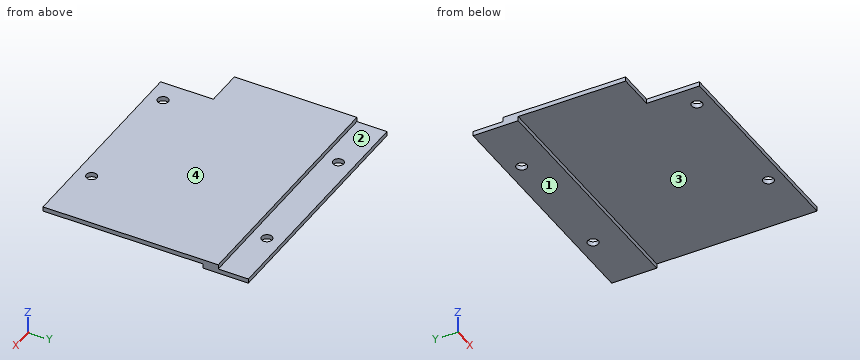
Solid Edge part; units mm, degrees
sketch "Sketch1" plane through (0, 0, 0) normal (0, 0, 1) x (1, 0, 0)
  line L0 (-82.5, -68.15) -> (82.5, -68.15)
  line L1 (82.5, -68.15) -> (82.5, 68.15)
  line L2 (82.5, 68.15) -> (-82.5, 68.15)
  line L3 (-82.5, 68.15) -> (-82.5, -68.15)
  dimension "D1" = 82.5
  dimension "D2" = 82.5
extrude "Extrusionsausprägung_1" add sketch "Sketch1" along normal blind 3
sketch "Sketch2" plane through (0, 0, 3) normal (0, 0, 1) x (1, 0, 0)
  circle A0 centre (-42.5, 58.15) radius 3.5
  circle A1 centre (42.5, 58.15) radius 3.5
  circle A2 centre (42.5, -58.15) radius 3.5
  circle A3 centre (-42.5, -58.15) radius 3.5
  dimension "D1" = 42.5
extrude "Extrusionsausschnitt_1" cut sketch "Sketch2" against normal blind 245.2559
sketch "Sketch3" plane through (0, 0, 3) normal (0, 0, 1) x (1, 0, 0)
  line L0 (-82.5, -68.15) -> (-57.5, -68.15)
  line L1 (-57.5, -68.15) -> (-57.5, -33.15)
  line L2 (-57.5, -33.15) -> (-82.5, -33.15)
  line L3 (-82.5, -33.15) -> (-82.5, -68.15)
  dimension "D1" = 57.5
  dimension "D2" = 57.5
extrude "Cutout1" cut sketch "Sketch3" against normal through all
sketch "Sketch4" plane through (0, 0, 0) normal (0, 0, -1) x (-1, 0, 0)
  line L0 (-82.5, 68.15) -> (82.5, 68.15)
  line L1 (82.5, 68.15) -> (82.5, 38.15)
  line L2 (82.5, 38.15) -> (-82.5, 38.15)
  line L3 (-82.5, 38.15) -> (-82.5, 68.15)
  dimension "D1" = 82.5
  dimension "D2" = 82.5
extrude "Extrusionsausprägung_2" add sketch "Sketch4" along normal blind 3
sketch "Sketch5" plane through (0, 0, 3) normal (0, 0, 1) x (1, 0, 0)
  circle A0 centre (-42.5, 58.15) radius 3.5
  circle A1 centre (42.5, 58.15) radius 3.5
extrude "Cutout2" cut sketch "Sketch5" against normal through all
sketch "Sketch6" plane through (-82.5, 17.5, 0) normal (-1, 0, 0) x (0, 1, 0)
  line L0 (50.65, 0) -> (30.65, 0)
  line L1 (30.65, 0) -> (30.65, -3)
  line L2 (30.65, -3) -> (50.65, -3)
  line L3 (50.65, -3) -> (50.65, 0)
  dimension "D1" = 30.65
  dimension "D2" = 50.65
extrude "Cutout3" cut sketch "Sketch6" against normal through all
properties material "Nylon, allgemein"
Work out the finished part from the listing and answer in its coordinate system (mm). Face numbers are marked on the shaded views. A direction names the side the tool comes from. Round coordinates to 2 decimals unless told otherwise and drop trailing zeros. Loops run counter-clockwise (first coordinate to the right, second up) from the corner with the lowest first, then second, coordinate; pieces in that order, holes last. Notation, with made-up numbers: (12, 24.25) -> (59, 24.25) arc R18 cw to (59, 49.25) -> close; hole circle Ø7 at (61, -33.5). An arc over 180 degrees is marked (long way). Use one line per item in the form item = value.
(1) For a pull along Z with two mould halves and no side action, classify the marked faces 3 and 4 as released by +Z, released by -Z, zero draft, split by the parting line, or undercut.
Answer list:
face_3 = released by -Z
face_4 = released by +Z
(2) Find section A-A on y = -58.15. Give the vertices of the cut face in (x, z).
Answer list:
outline = (-57.5, 0) -> (-46, 0) -> (-46, 3) -> (-57.5, 3) -> close; (-39, 0) -> (39, 0) -> (39, 3) -> (-39, 3) -> close; (46, 0) -> (82.5, 0) -> (82.5, 3) -> (46, 3) -> close
(3) Find section C-C on z = 1.65. Give the vertices of the cut face in (x, y), then the cut area to 3 significant figures.
Answer list:
outline = (-82.5, -33.15) -> (-57.5, -33.15) -> (-57.5, -68.15) -> (82.5, -68.15) -> (82.5, 48.15) -> (-82.5, 48.15) -> close; hole circle Ø7 at (-42.5, -58.15); hole circle Ø7 at (42.5, -58.15)
area = 18,200 mm2
(4) Find section D-D on x = 0.5. Give the vertices of the cut face in (y, z).
Answer list:
outline = (-68.15, 0) -> (38.15, 0) -> (38.15, -3) -> (68.15, -3) -> (68.15, 0) -> (48.15, 0) -> (48.15, 3) -> (-68.15, 3) -> close
(5) A tool of negligible diameter and unlimited length cuts with its end or side. For the marked faces 1 and 2, from which of +Z, -Z, +X, -X, +Y, -Y can it reach the whole face along a straight path? Write none if from no direction.
Answer list:
face_1 = -Z, +X, -X, +Y, -Y
face_2 = +Z, +X, -X, +Y
(6) Find section B-B on x = -42.5. Give the vertices of the cut face in (y, z), then the cut area to 3 significant figures.
Answer list:
outline = (-68.15, 0) -> (-61.65, 0) -> (-61.65, 3) -> (-68.15, 3) -> close; (-54.65, 0) -> (38.15, 0) -> (38.15, -3) -> (54.65, -3) -> (54.65, 0) -> (48.15, 0) -> (48.15, 3) -> (-54.65, 3) -> close; (61.65, -3) -> (68.15, -3) -> (68.15, 0) -> (61.65, 0) -> close
area = 397 mm2
(7) Straight lines are drawn through the part: line 1 (Y direction, x = -42.5, z = 1.1); line 2 (Y direction, x = -42.5, z = -1.55); line 3 (Z direction, x = -3, y = 55). For each, find the intervals that lie inside material, in ascending order.
Answer list:
line_1 = -68.15 to -61.65, -54.65 to 48.15
line_2 = 38.15 to 54.65, 61.65 to 68.15
line_3 = -3 to 0
(8) Flat-ended cylindrical pins translate along their axes: P1, Ø16, axis at x = -27.5, y = 56, coming from the +Z side; P2, Ø2.5, axis at y = -57.5, z = 1.5, coming from the -X side; P3, Ø2.5, axis at x = -71.5, z = 1.5, coming from the -Y side; P4, Ø2.5, axis at x = -6.5, z = 1.5, coming from the +Y side. Find the tip coordinate at first contact, or state that the pin passes through.
Answer list:
P1 = 3
P2 = -57.5
P3 = -33.15
P4 = 48.15
